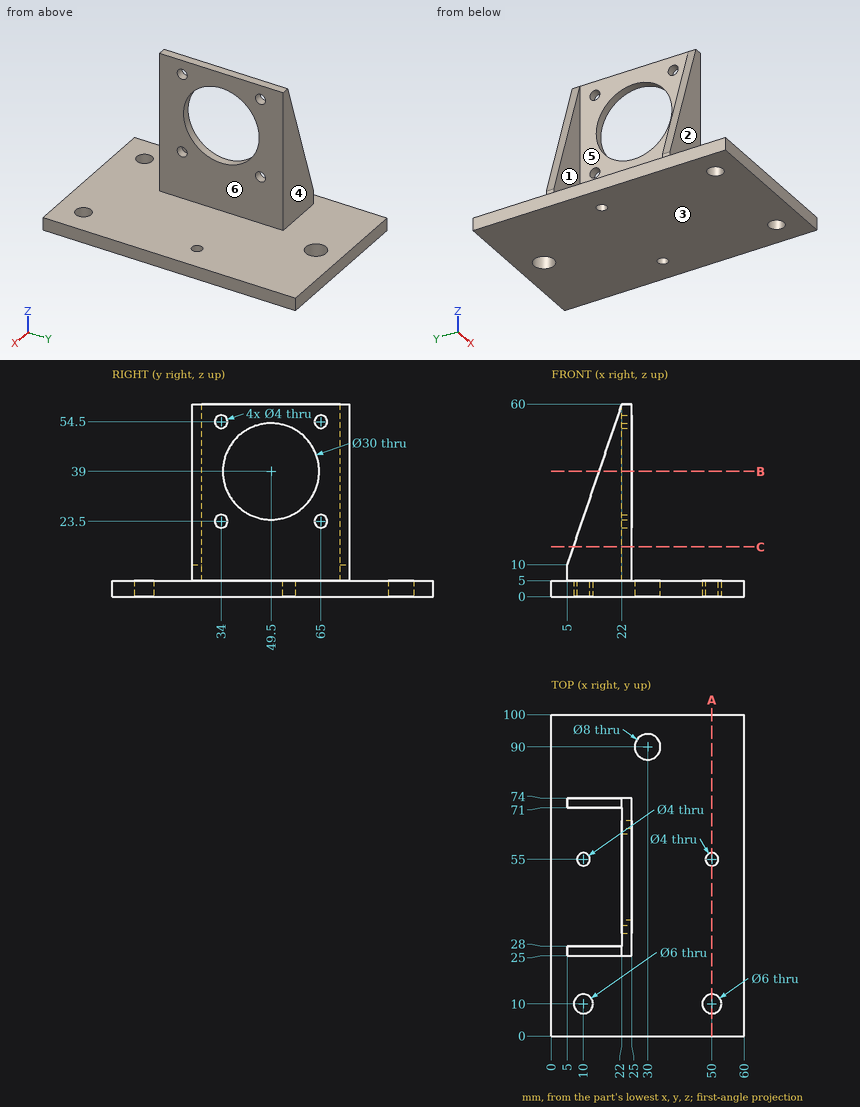
The drawing under review shows one solid part. Ordinate dimensions are in mm from its lowest x, y, z. A direction names the side the tool comes from. Give positions to 0.01 mm unless a question says otherwise; leave off trailing zeros. Write each loop counter-clockwise with the first axis right and the second up, starting at its lowest first coordinate (ties: lowest second). Pieces come first, ordered by that corner, then holes. Notation, with made-up numbers: (-7, 8.5) -> (51, 8.5) arc R14 cw to (51, 17.5) -> close; hole circle Ø10 at (54, 54.25). An arc over 180 degrees is marked (long way). Answer in a Markdown table with one row per item.
(1) For the marked faces 4, 5 and 6, list the 3-axis set-ups (+Z, -Z, +X, -X, +Y, -Y) from which the entire face can be reached by the end or side of a thin tool; tool diameter is ignored.
Results:
| item | result |
|---|---|
| face 4 | +Z, +X, -X, +Y |
| face 5 | +Z, -X |
| face 6 | +Z, +X, +Y, -Y |
(2) Mouldability with a two-part tool opening along Y and no side actions: class the marked faces 1, 2 and 3 as +Y half, -Y half, draft (parallel to the pull), parting line (faces both ways), or undercut.
Results:
| item | result |
|---|---|
| face 1 | undercut |
| face 2 | -Y half |
| face 3 | draft |
(3) Consider section A-A (x = 50). State the section outline as (y, z) points.
Results:
| item | result |
|---|---|
| outline | (0, 0) -> (7, 0) -> (7, 5) -> (0, 5) -> close; (13, 0) -> (53, 0) -> (53, 5) -> (13, 5) -> close; (57, 0) -> (100, 0) -> (100, 5) -> (57, 5) -> close |
(4) Consider section C-C (z = 15.5). State the section outline as (x, y) points.
Results:
| item | result |
|---|---|
| outline | (6.87, 25) -> (25, 25) -> (25, 74) -> (6.87, 74) -> (6.87, 71) -> (22, 71) -> (22, 28) -> (6.87, 28) -> close |
(5) Consider section B-B (z = 39). State the section outline as (x, y) points.
Results:
| item | result |
|---|---|
| outline | (14.86, 25) -> (25, 25) -> (25, 34.5) -> (22, 34.5) -> (22, 28) -> (14.86, 28) -> close; (14.86, 71) -> (22, 71) -> (22, 64.5) -> (25, 64.5) -> (25, 74) -> (14.86, 74) -> close |
(6) To check wall thickness, follow probe 1 along Y at (x, z) = (10, 3.95); probe 2 along Z at (x, y) = (24, 34); probe 3 along Y at (x, z) = (11.5, 28). State the ranges of each line that lie inside material, in increasing order.
Results:
| item | result |
|---|---|
| probe 1 | 0 to 7, 13 to 53, 57 to 100 |
| probe 2 | 0 to 21.5, 25.5 to 52.5, 56.5 to 60 |
| probe 3 | 25 to 28, 71 to 74 |
(7) Clearance check with flat-ended pins moving along their axes: pin 1 (6.5 mm diameter, centred on y = 34, z = 54.5, fed in from -X); pin 2 (4 mm diameter, centred on x = 33.5, y = 51.5, fed in from -Z); pin 3 (18.5 mm diameter, centred on x = 14.5, z = 41.5, fed in from -Y); pin 4 (3 mm diameter, centred on x = 10, y = 55, fed in from -Z). State where each tip first meets the part, or that it passes through.
Results:
| item | result |
|---|---|
| pin 1 | x = 22 |
| pin 2 | z = 0 |
| pin 3 | y = 25 |
| pin 4 | through |
